from build123d import *

# Parameters (mm, degrees)
SKETCH1_R               = 7.5
BOSS_EXTRUDE1_DEPTH     = 5
SKETCH2_R               = 8.5
BOSS_EXTRUDE2_DEPTH     = 2
SKETCH3_R               = 7.5
BOSS_EXTRUDE3_DEPTH     = 35
SKETCH4_R               = 4
CUT_EXTRUDE1_DEPTH      = 44.686382318
CUT_EXTRUDE3_REACH      = 47.741
CUT_EXTRUDE3_END_RADIUS = 4
SKETCH7_R               = 1
CUT_EXTRUDE6_START      = -14
SKETCH9_R               = 7.5
SKETCH9_R_2             = 7
CUT_EXTRUDE6_DEPTH      = 14
FILLET1_R               = 0.8
SKETCH10_W              = 3
SKETCH10_H              = 3
CUT_EXTRUDE7_DEPTH      = 28
SKETCH12_W              = 5
SKETCH12_H              = 5
CUT_EXTRUDE8_DEPTH      = 18.5


with BuildPart() as part:
    # Sketch1 → Boss-Extrude1 (new body)
    with BuildSketch(Plane(origin=(0, 0, 0), x_dir=(0, 0, -1), z_dir=(1, 0, 0))):
        Circle(SKETCH1_R)
    extrude(amount=BOSS_EXTRUDE1_DEPTH)

    # Sketch2 → Boss-Extrude2 (add)
    with BuildSketch(Plane(origin=(5, 0, 0), x_dir=(0, 0, -1), z_dir=(1, 0, 0))):
        Circle(SKETCH2_R)
    extrude(amount=BOSS_EXTRUDE2_DEPTH)

    # Sketch3 → Boss-Extrude3 (add)
    with BuildSketch(Plane(origin=(7, 0, 0), x_dir=(0, 0, -1), z_dir=(1, 0, 0))):
        Circle(SKETCH3_R)
    extrude(amount=BOSS_EXTRUDE3_DEPTH)

    # Sketch4 → Cut-Extrude1 (cut, through all)
    with BuildSketch(Plane.ZY):
        Circle(SKETCH4_R)
    extrude(amount=-CUT_EXTRUDE1_DEPTH, mode=Mode.SUBTRACT)

    # Cut-Extrude3: up to this cylinder (the profile starts outside it)
    cut_extrude3_end = Plane(origin=(12, 0, 0), z_dir=(-1, 0, 0)) * Cylinder(CUT_EXTRUDE3_END_RADIUS, 104.482, mode=Mode.PRIVATE)
    # Sketch7 → Cut-Extrude3 (cut, up to the surface)
    with BuildSketch(Plane(origin=(0, 7.5, 0), x_dir=(1, 0, 0), z_dir=(0, 1, 0)), mode=Mode.PRIVATE) as cut_extrude3_sk1:
        with Locations(Location((12, 0, 0), (0, 0, 270))):
            Circle(SKETCH7_R)
    cut_extrude3_tool1 = extrude(cut_extrude3_sk1.sketch, amount=-CUT_EXTRUDE3_REACH, mode=Mode.PRIVATE) - cut_extrude3_end
    add(cut_extrude3_tool1.solids().sort_by_distance((12, 7.5, 0))[0], mode=Mode.SUBTRACT)

    # Sketch9 → Cut-Extrude6 (cut)
    with BuildSketch(Plane(origin=(42, 0, 0), x_dir=(0, 0, -1), z_dir=(1, 0, 0)).offset(CUT_EXTRUDE6_START)):
        Circle(SKETCH9_R)
        Circle(SKETCH9_R_2, mode=Mode.SUBTRACT)
    extrude(amount=CUT_EXTRUDE6_DEPTH, mode=Mode.SUBTRACT)

    # Fillet1
    # the kernel refuses this fillet: 0.8 mm, written as the material it adds along each edge
    with BuildSketch(Plane(origin=(28, 0, 0), x_dir=(0, 0, -1), z_dir=(0, -1, 0))) as fillet1_piece_1:
        with BuildLine():
            CenterArc((7.8, 0.741619849), FILLET1_R, 180, 67.975687163)
            Line((7, 0.741619849), (6.984, 0.741619849))
            Line((6.984, 0.741619849), (6.984, 0))
            Line((6.984, 0), (7, -0.016))
            ThreePointArc((7, -0.016), (7.25, -0.016), (7.494, -0.014832397))
            Line((7.494, -0.014832397), (7.5, 0))
        make_face()
    revolve(axis=Axis((28, 0, 0), (1, 0, 0)))

    # Sketch10 → Cut-Extrude7 (cut)
    with BuildSketch(Plane.ZY):
        with Locations((0, 4)):
            Rectangle(SKETCH10_W, SKETCH10_H)
    extrude(amount=-CUT_EXTRUDE7_DEPTH, mode=Mode.SUBTRACT)

    # Sketch12 → Cut-Extrude8 (cut)
    with BuildSketch(Plane(origin=(27, 0, 0), x_dir=(0, 0, -1), z_dir=(1, 0, 0))):
        with Locations((0, -7.5)):
            Rectangle(SKETCH12_W, SKETCH12_H)
    extrude(amount=-CUT_EXTRUDE8_DEPTH, mode=Mode.SUBTRACT)


solid = part.part
The listing builds one solid part. Answer for the finished solid, in the listing's coordinates (mm). A direction names the side the tool comes from. Give positions to 0.01 mm unless a question says otherwise; leave off trailing zeros. Order: outer loops, then holes, each group sorted by start corner. A loop starts at its lowest first (then second) coordinate and runs counter-clockwise, first axis right, second up. Notation, with made-up numbers: (24.25, 34) - (68.25, 34) arc R19 ccw to (68.25, 43) - close; hole circle Ø1 at (46.5, -22). An arc over 180 degrees is marked (long way). One line per item, written item: value. Start each with the question number.
1) A cutting plane is placed at A-A on z = 0. State how many separate pieces and enclosed holes the cut face has, then the cut area to 3 significant figures.
2) A tool of negligible diameter and unlimited length cuts with its end or side. For faces 4 (the face through (27, -6, 0)), 5 (the face through (17.353, 6.324, -4.032)), 6 (the face through (28, 5, 0)), from which of +Z, -Z, +X, -X, +Y, -Y can it reach the whole face along a straight path? Write none if from no direction.
3) A cutting plane is placed at B-B on y = 0. Give the vertices of the cut face in (x, z).
4) A cutting plane is placed at D-D on x = 3. Give the vertices of the cut face in (y, z).
5) The mould has two halves that part along Y. Classify faces 1 (the face through (18, -5, 0)), 2 (the face through (8.5, -6, 0)), 3 (the face through (14, 5, -1.5)): released by +Y, released by -Y, zero draft, split by the parting line, or undercut.
6) Given pin 1 Ø4 at (x, z) = (14, 5) entering from -Y; pin 2 Ø2.5 at (x, z) = (10.5, 0) entering from -Y; pin 3 Ø1.4 at (x, y) = (15, 5) entering from -Z; pin 4 Ø6.5 at (y, z) = (0, 0) entering from -X, each flat-ended and moving along its own axis, determine where each tip first touches the part or whether it passes through.
7) A cutting plane is placed at C-C on x = 9. Give the vertices of the cut face in (y, z).
8) Find the intervals of material crossed by L1, parallel to Y at x = 21.5, z = 0; L2, parallel to Z at x = 17, y = 0.25; L3, parallel to X at y = 6.15, z = 0, in increasing order.
Answer sheet:
1. separate pieces: 3
1. enclosed holes: 0
1. area: 192 mm2
2. face 4: -Y
2. face 5: +X
2. face 6: -X
3. outline: (0, -7.5) - (5, -7.5) - (5, -8.5) - (7, -8.5) - (7, -7.5) - (28, -7.5) arc R0.8 cw to (28.74, -7) - (42, -7) - (42, -4) - (0, -4) - close; (0, 4) - (42, 4) - (42, 7) - (28.74, 7) arc R0.8 cw to (28, 7.5) - (7, 7.5) - (7, 8.5) - (5, 8.5) - (5, 7.5) - (0, 7.5) - close
4. outline: circle Ø15 at (0, 0); hole (3.71, -1.5) - (5.5, -1.5) - (5.5, 1.5) - (3.71, 1.5) arc R4 ccw (long way) to start
5. face 1: released by -Y
5. face 2: zero draft
5. face 3: undercut
6. pin 1: stops at y = -6.87
6. pin 2: stops at y = -5
6. pin 3: stops at z = -6.14
6. pin 4: passes through
7. outline: (-7.07, -2.5) arc R7.5 ccw (long way) to (-7.07, 2.5) - (-5, 2.5) - (-5, -2.5) - close; hole (3.71, -1.5) - (5.5, -1.5) - (5.5, 1.5) - (3.71, 1.5) arc R4 ccw (long way) to start
8. L1: y = -5 to -4, 5.5 to 7.5
8. L2: z = -7.5 to -3.99, 3.99 to 7.5
8. L3: x = 0 to 11, 13 to 42
